Input: part model. Units: mm. Frame: model coordinates. Face numbers are marked on the shaded views. A direction names the side the tool comes from. Coordinates: 2 decimals unless noted, no trailing zeros. Write each loop counter-clockwise with the first axis right and the second up, starting at its lowest first coordinate (ties: lowest second). Pieces come first, ordered by that corner, then holes. Notation, with made-up numbers: (-27, 30) - (16, 30) arc R21 ccw to (16, 59) - close; hole circle Ø2 at (40.25, 3.5). An arc over 180 degrees is marked (long way). Put each result on its own line as item: value. Start each with the question number.
1. Pull-direction query (Y, two-part tool) for the marked faces 1, 2, 3 and 4; classes: released by +Y, released by -Y, zero draft, split by the parting line, or undercut.
2. Cut plane A-A, the plane y = 0. Return loops of the section in (x, z) (3 decimals).
3. Access query for the marked faces 5 and 6. Directions: +Z, -Z, +X, -X, +Y, -Y. A direction counts if a zero-diameter tool reaches every point of the face in a straight line with its end or side. Return the directions, or none.
4. Pin query (flat end, axial travel): pin 1 (5 mm diameter, centred on x = 0, y = 0, fed in from -Z); pin 2 (2 mm diameter, centred on y = 6.5, z = -2, fed in from -X). Return the tip coordinate at first contact, or that it passes through.
5. Line query: line 1 (Y direction, x = 0, z = -1.9); line 2 (Z direction, x = -7.75, y = -2.5); line 3 (X direction, y = -2.25, z = -3.65). Output: solid intervals per line, ascending.
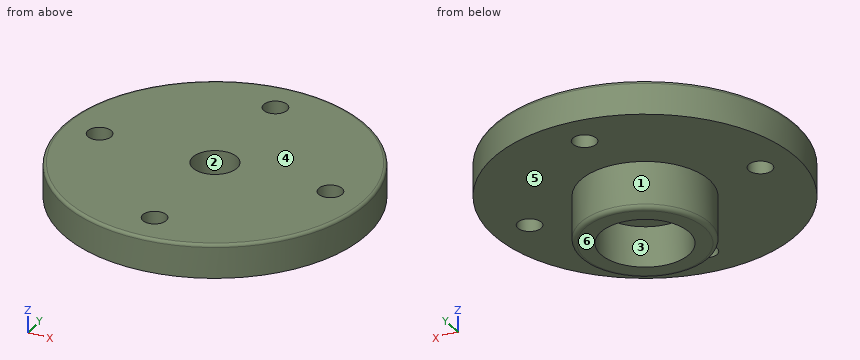
from build123d import *

# Parameters (mm, degrees)
SKETCH1_R           = 10.3
BOSS_EXTRUDE1_DEPTH = 2.3
SKETCH2_R           = 4.375
BOSS_EXTRUDE2_DEPTH = 3.2
SKETCH3_R           = 3
CUT_EXTRUDE1_DEPTH  = 2.75
SKETCH4_R           = 1.5
CUT_EXTRUDE2_DEPTH  = 16.570163776
SKETCH12_R          = 0.8
CUT_EXTRUDE10_DEPTH = 15.913752043
FILLET2_R           = 0.2
FILLET3_R           = 0.3


with BuildPart() as part:
    # Sketch1 → Boss-Extrude1 (new body)
    with BuildSketch(Plane(origin=(0, 0, -2.5), x_dir=(-1, 0, 0), z_dir=(0, 0, -1))):
        with Locations(Location((0, 0, 0), (0, 0, 180))):
            Circle(SKETCH1_R)
    extrude(amount=-BOSS_EXTRUDE1_DEPTH)

    # Sketch2 → Boss-Extrude2 (add)
    with BuildSketch(Plane(origin=(0, 0, -2.5), x_dir=(-1, 0, 0), z_dir=(0, 0, -1))):
        Circle(SKETCH2_R)
    extrude(amount=BOSS_EXTRUDE2_DEPTH)

    # Sketch3 → Cut-Extrude1 (cut)
    with BuildSketch(Plane(origin=(0, 0, -5.7), x_dir=(-1, 0, 0), z_dir=(0, 0, -1))):
        with Locations(Location((0, 0, 0), (0, 0, 180))):
            Circle(SKETCH3_R)
    extrude(amount=-CUT_EXTRUDE1_DEPTH, mode=Mode.SUBTRACT)

    # Sketch4 → Cut-Extrude2 (cut, through all)
    with BuildSketch(Plane.XY.offset(-0.2)):
        Circle(SKETCH4_R)
    extrude(amount=-CUT_EXTRUDE2_DEPTH, mode=Mode.SUBTRACT)

    # Sketch12 → Cut-Extrude10 (cut, through all)
    with BuildSketch(Plane(origin=(0, 0, -2.5), x_dir=(-1, 0, 0), z_dir=(0, 0, -1))):
        with Locations(Location((0, 7.8, 0), (0, 0, 180))):
            Circle(SKETCH12_R)
        with Locations(Location((7.8, 0, 0), (0, 0, 180))):
            Circle(SKETCH12_R)
        with Locations(Location((0, -7.8, 0), (0, 0, 180))):
            Circle(SKETCH12_R)
        with Locations(Location((-7.8, 0, 0), (0, 0, 180))):
            Circle(SKETCH12_R)
    extrude(amount=-CUT_EXTRUDE10_DEPTH, mode=Mode.SUBTRACT)

    # Fillet2
    fillet2_edges = [part.edges().sort_by_distance(p)[0] for p in [
        (-10.3, 0, -0.2),
    ]]
    fillet(fillet2_edges, radius=FILLET2_R)

    # Fillet3
    fillet3_edges = [part.edges().sort_by_distance(p)[0] for p in [
        (4.375, 0, -5.7),
    ]]
    fillet(fillet3_edges, radius=FILLET3_R)


solid = part.part
Report:
1. face 1: split by the parting line
1. face 2: undercut
1. face 3: undercut
1. face 4: zero draft
2. outline: (-10.3, -2.5) - (-8.6, -2.5) - (-8.6, -0.2) - (-10.1, -0.2) arc R0.2 ccw to (-10.3, -0.4) - close; (-7, -2.5) - (-4.375, -2.5) - (-4.375, -5.4) arc R0.3 ccw to (-4.075, -5.7) - (-3, -5.7) - (-3, -2.95) - (-1.5, -2.95) - (-1.5, -0.2) - (-7, -0.2) - close; (1.5, -2.95) - (3, -2.95) - (3, -5.7) - (4.075, -5.7) arc R0.3 ccw to (4.375, -5.4) - (4.375, -2.5) - (7, -2.5) - (7, -0.2) - (1.5, -0.2) - close; (8.6, -2.5) - (10.3, -2.5) - (10.3, -0.4) arc R0.2 ccw to (10.1, -0.2) - (8.6, -0.2) - close
3. face 5: -Z
3. face 6: -Z, +X, -X, +Y, -Y
4. pin 1: stops at z = -2.95
4. pin 2: stops at x = -8.71
5. line 1: y = -10.3 to -8.6, -7 to -1.5, 1.5 to 7, 8.6 to 10.3
5. line 2: z = -2.5 to -0.2
5. line 3: x = -3.75 to -1.98, 1.98 to 3.75
